Can you work these out from the model? Positions are in its coordinate system, mm. A direction names the side the tool comes from. Coordinates: 2 decimals unless noted, no trailing zeros. Loops run counter-clockwise (first coordinate to the right, second up) from the corner with the lowest first, then second, coordinate; pieces in that order, holes last. Notation, with made-up numbers: (35.25, -8) -> (71.25, -8) arc R32 cw to (71.25, 18) -> close; hole circle Ø7 at (34, 7). An arc over 180 degrees is marked (long way). Put each result on its own line as item: value. Start each with the question number.
Item 1: We'd pull the mould along X, two halves only. Please class faces 1 (the cylindrical face through (-6.386, 4.425, 0.986)), 2 (the flat face through (0, -2, 2)), 3 (the cylindrical face through (-0.867, 3.905, -1.479)): pulls with the +X half, pulls with the -X half, needs draft (parallel to the pull), parting line crosses it, or undercut.
Item 2: If we section it at C-C on x = 5: Please give me the cut outline in (y, z), plus the area to 3 significant figures.
Item 3: Please list where these lines run through material, in increasing order: L1, parallel to Y at x = -4, z = 1; L2, parallel to X at y = 0, z = -1.15; L3, parallel to Z at x = -8.25, y = -3.25. Write a range as from..to.
Item 4: If we section it at A-A on y = 0: Please give me the cut outline in (x, z), plus the area to 3 significant figures.
Item 5: If we section it at B-B on z = 0.25: Please give me the cut outline in (x, y), plus the area to 3 significant figures.
Item 6: Will these pins go through, and if not, where does the flat tip stop? P1, Ø2, axis at y = 6.5, z = -2, coming from the -X side; P2, Ø4, axis at x = -5, y = -5, coming from the -Z side; P3, Ø1, axis at x = -3.5, z = 1.5, coming from the -Y side; P4, Ø1, axis at y = -6.5, z = 1, coming from the +X side.
Item 7: If we section it at D-D on y = -4.25: Please give me the cut outline in (x, z), plus the area to 3 significant figures.
Item 8: For faces 4 (the cylindrical face through (-5.806, -3.735, 0.986)), 5 (the cylindrical face through (-0.54, 2.44, -1.48)), which set-ups out of +Z, -Z, +X, -X, +Y, -Y let a thin tool reach every point of the face, with its end or its side?
```python
from build123d import *

# Parameters (mm, degrees)
F0_R     = 10
F0_R_2   = 1.5
F1_DEPTH = 2
F3_D     = 3
F4_R     = 4
F4_R_2   = 2.5
F5_DEPTH = 3


# Not quite as in the source:
# - a feature names something its author has since deleted; it is built from what else it names


with BuildPart() as f1:
    # F0 (on Top) → F1 (new body)
    with BuildSketch(Plane.XY):
        Circle(F0_R)
        Circle(F0_R_2, mode=Mode.SUBTRACT)
    extrude(amount=F1_DEPTH)

    # F3 (through all)
    with Locations(Plane.XY.offset(2)):
        with Locations((-5, 5), (5, 5), (5, -5), (-5, -5)):
            Hole(F3_D / 2)

    # F4 (on face) → F5 (join)
    with BuildSketch(Plane(origin=(0, 0, 0), x_dir=(1, 0, 0), z_dir=(0, 0, -1))):
        Circle(F4_R)
        Circle(F4_R_2, mode=Mode.SUBTRACT)
    extrude(amount=F5_DEPTH)


solid = f1.part
```
Solutions:
1. face 1: undercut
1. face 2: needs draft
1. face 3: parting line crosses it
2. outline: (-8.66, 0) -> (-6.5, 0) -> (-6.5, 2) -> (-8.66, 2) -> close; (-3.5, 0) -> (3.5, 0) -> (3.5, 2) -> (-3.5, 2) -> close; (6.5, 0) -> (8.66, 0) -> (8.66, 2) -> (6.5, 2) -> close
2. area: 22.6 mm^2
3. L1: -9.17..-6.12, -3.88..3.88, 6.12..9.17
3. L2: -4..-2.5, 2.5..4
3. L3: 0..2
4. outline: (-10, 0) -> (-4, 0) -> (-4, -3) -> (-2.5, -3) -> (-2.5, 0) -> (-1.5, 0) -> (-1.5, 2) -> (-10, 2) -> close; (1.5, 0) -> (2.5, 0) -> (2.5, -3) -> (4, -3) -> (4, 0) -> (10, 0) -> (10, 2) -> (1.5, 2) -> close
4. area: 43.0 mm^2
5. outline: circle Ø20 at (0, 0); hole circle Ø3 at (-5, -5); hole circle Ø3 at (-5, 5); hole circle Ø3 at (0, 0); hole circle Ø3 at (5, -5); hole circle Ø3 at (5, 5)
5. area: 279 mm^2
6. P1: through
6. P2: z = 0
6. P3: y = -9.54
6. P4: x = 8
7. outline: (-9.05, 0) -> (-6.3, 0) -> (-6.3, 2) -> (-9.05, 2) -> close; (-3.7, 0) -> (3.7, 0) -> (3.7, 2) -> (-3.7, 2) -> close; (6.3, 0) -> (9.05, 0) -> (9.05, 2) -> (6.3, 2) -> close
7. area: 25.8 mm^2
8. face 4: +Z, -Z
8. face 5: -Z
